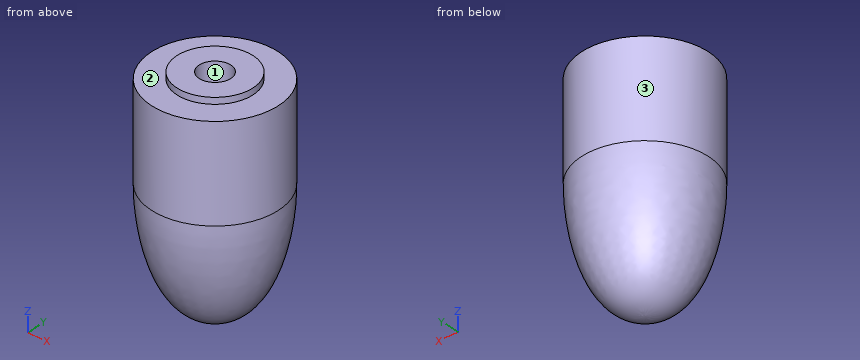
```python
from build123d import *

# Parameters (mm, degrees)
F2_R     = 2.5
F3_DEPTH = 25
F5_ANGLE = 90


with BuildPart() as f1:
    # F0 (on Front) → F1 (revolve)
    with BuildSketch(Plane.XZ):
        with BuildLine():
            Line((-8.5, 0), (0, 0))
            Line((0, 0), (26.5, 0))
            add(Edge.make_bspline(
                [(7.5, 10), (14.95356, 10), (26.5, 7.45356), (26.5, 0)],
                knots=[0, 0, 0, 0, 21.470911, 21.470911, 21.470911, 21.470911], degree=3))
            Line((7.5, 10), (-7.5, 10))
            Line((-7.5, 10), (-7.5, 6))
            Line((-7.5, 6), (-8.5, 6))
            Line((-8.5, 6), (-8.5, 0))
        make_face()
    revolve(axis=Axis((13.25, 0, 0), (1, 0, 0)))

    # F2 (on face) → F3 (cut)
    with BuildSketch(Plane(origin=(-8.5, 0, 0), x_dir=(0, -1, 0), z_dir=(-1, 0, 0))):
        Circle(F2_R)
    extrude(amount=-F3_DEPTH, mode=Mode.SUBTRACT)


with BuildPart() as f1_1:
    # F5: moved
    add(f1.part.rotate(Axis((0, 12.53504, 0), (0, 1, 0)), F5_ANGLE))


solid = f1_1.part
```
The model under review builds one solid part; all positions refer to its coordinate system, in mm. Face numbers are marked on the shaded views. Round coordinates to 2 decimals unless told otherwise and drop trailing zeros. Write each loop counter-clockwise with the first axis right and the second up, starting at its lowest first coordinate (ties: lowest second). Pieces come first, ordered by that corner, then holes. Notation, with made-up numbers: (22, 42) - (55, 42) arc R9 cw to (55, 46) - close; hole circle Ø4 at (-30, 44). An arc over 180 degrees is marked (long way). Use one line per item in the form item = value.
Q1. Consider section A-A (z = 4.5). State the section outline as (x, y) points, and give its area (3 significant figures).
Answer key:
outline = circle Ø20 at (0, 0); hole circle Ø5 at (0, 0)
area = 295 mm2
Q2. Draft analysis for pull direction Y (two halves, no side actions). For the marked faces 1, 2 and 3, state which applies: +Y half, -Y half, draft (parallel to the pull), parting line (faces both ways), or undercut.
Answer key:
face_1 = undercut
face_2 = draft
face_3 = parting line
Q3. Insertion check: pin 1 Ø1.5 at (x, y) = (-2, 3.5) entering from -Z; pin 2 Ø3 at (x, z) = (-0.5, -10) entering from -Y; pin 3 Ø1.5 at (x, y) = (0, -1) entering from +Z. Each pin has a flat end and moves straight along its axis. Give the tip position at first contact, or say it passes through.
Answer key:
pin_1 = -25.64
pin_2 = -9.98
pin_3 = -16.5
Q4. For line 1 (X direction, y = 0, z = -2.25); line 2 (X direction, y = -1.5, z = -14); line 3 (X direction, y = -6.75, z = -11.5), list the stretches that pass through material, from the lowest coordinate up. Write a range as [from, to].
Answer key:
line_1 = [-10, -2.5], [2.5, 10]
line_2 = [-9.3, -2], [2, 9.3]
line_3 = [-7.07, 7.07]
